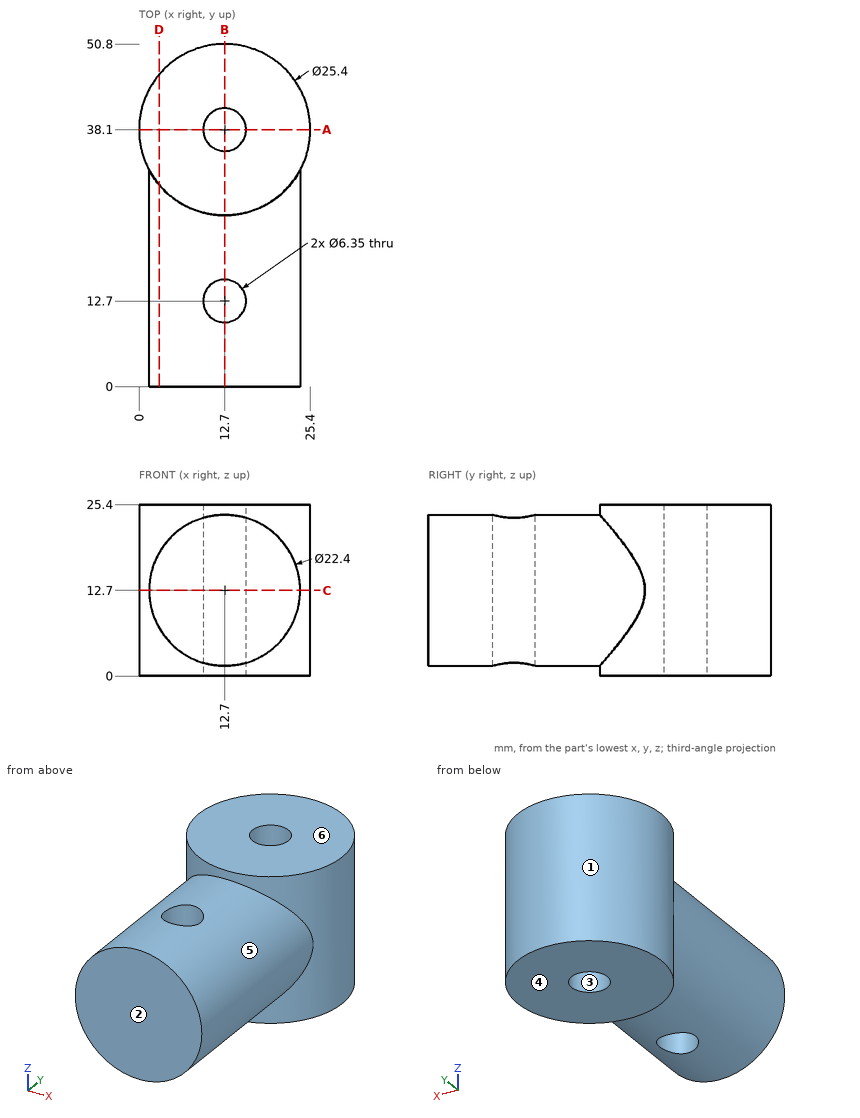
Verification items for this drawing (mm, ordinates from the low corner). A direction names the side the tool comes from. Give positions to 0.01 mm unless a question says otherwise; leave off trailing zeros. Write each loop counter-clockwise with the first axis right and the second up, starting at its lowest first coordinate (ties: lowest second). Pieces come first, ordered by that corner, then holes.
1) Release check for a two-part mould opening along Y. For the marked faces 1, 2, 3 and 4 record: released by +Y, released by -Y, zero draft, split by the parting line, or undercut.
Values follow:
face 1: split by the parting line
face 2: released by -Y
face 3: undercut
face 4: zero draft
2) Cross-section at D-D (x = 3). Record the boundary of the cut face in (y, z), plus the area to 3 significant figures.
Values follow:
outline: (0, 7.1) - (29.9, 7.1) - (29.9, 0) - (46.3, 0) - (46.3, 25.4) - (29.9, 25.4) - (29.9, 18.3) - (0, 18.3) - close
area: 751 mm2
3) Cross-section at B-B (x = 12.7). Record the boundary of the cut face in (y, z) (3 decimals).
Values follow:
outline: (0, 1.5) - (9.525, 1.5) - (9.525, 23.9) - (0, 23.9) - close; (15.875, 1.5) - (25.4, 1.5) - (25.4, 0) - (34.925, 0) - (34.925, 25.4) - (25.4, 25.4) - (25.4, 23.9) - (15.875, 23.9) - close; (41.275, 0) - (50.8, 0) - (50.8, 25.4) - (41.275, 25.4) - close
4) Set-up check for the marked faces 5 and 6: record each of +Z, -Z, +X, -X, +Y, -Y from which the full face is reachable in a straight line by a thin tool's end or side.
Values follow:
face 5: -Y
face 6: +Z, +X, -X, +Y, -Y
5) Cross-section at A-A (y = 38.1). Record the boundary of the cut face in (x, z) (3 decimals).
Values follow:
outline: (0, 0) - (9.525, 0) - (9.525, 25.4) - (0, 25.4) - close; (15.875, 0) - (25.4, 0) - (25.4, 25.4) - (15.875, 25.4) - close
6) Thickness scan on line 1 (Y direction, x = 12.7, z = 9.5) (3 decimals); line 2 (X direction, y = 13.5, z = 13.5); line 3 (Z direction, x = 9, y = 6). Record the ranges inside material, lowest first.
Values follow:
line 1: y = 0 to 9.525, 15.875 to 34.925, 41.275 to 50.8
line 2: x = 1.53 to 9.63, 15.77 to 23.87
line 3: z = 2.13 to 23.27
7) Go/stop test with flat-tipped pins: pin 1 Ø12 at (x, y) = (5, 5.5) entering from +Z; pin 2 Ø1.5 at (x, z) = (11, 19.5) entering from +Y; pin 3 Ø2 at (y, z) = (36.5, 22) entering from +X. Record where each tip stops, or that it passes through.
Values follow:
pin 1: stops at z = 23.77
pin 2: stops at y = 50.76
pin 3: stops at x = 25.39
8) Cross-section at C-C (z = 12.7). Record the boundary of the cut face in (x, y) (3 decimals).
Values follow:
outline: (1.5, 0) - (23.9, 0) - (23.9, 32.113) arc R12.7 ccw (long way) to (1.5, 32.113) - close; hole circle Ø6.35 at (12.7, 12.7); hole circle Ø6.35 at (12.7, 38.1)
